Source: CAD feature listing. Evaluate the final solid. Frame: model axes, mm. A direction names the side the tool comes from. Give positions to 0.01 mm unless a question says otherwise; leave off trailing zeros. Write each loop counter-clockwise with the first axis right and the second up, starting at its lowest first coordinate (ties: lowest second). Pieces come first, ordered by that corner, then holes. Notation, with made-up numbers: (46.5, 80.25) -> (100.5, 80.25) arc R34 ccw to (100.5, 116.25) -> close; hole circle Ø11 at (60.5, 66.5). An arc over 180 degrees is marked (long way). Answer as a JSON object with one key per item and string values. Group by question number.
Item 1: Ray query, probe 1 along Y at (x, z) = (3.5, -11) (3 decimals); probe 2 along Z at (x, y) = (5.5, -1.25) (3 decimals); probe 3 along Y at (x, z) = (2.5, -16.5). Return the intervals inside material, ascending. Write a range as from..to.
Item 2: First-contact query: pin 1 Ø2 at (x, z) = (1.5, 6) entering from +Y (3 decimals); pin 2 Ø10 at (x, y) = (2, 9) entering from +Z (3 decimals). Flat tips, straight axial feed; report the tip coordinate or a pass-through.
Item 3: Access query for faces 4 (the face through (3.175, 2, -17)), 5 (the face through (9.525, -11, 2)), 6 (the face through (12.7, -10, -7)), 7 (the face through (-6, 3, -15.875)), 8 (the face through (0, -12.7, 0)). Directions: +Z, -Z, +X, -X, +Y, -Y. A direction counts if a zero-diameter tool reaches every point of the face in a straight line with its end or side. Return the directions, or none.
Item 4: Section query B-B on y = -1.5. Return the cut outline in (x, z) (3 decimals).
Item 5: Pull-direction query (X, two-part tool) for faces 1 (the face through (-12.7, -10, -7)), 2 (the face through (-0.07, -6.03, -17.44)), 3 (the face through (5, 0, -19.05)); classes: pulls with the +X half, pulls with the -X half, needs draft (parallel to the pull), parting line crosses it, or undercut.
Item 6: Section query A-A on x = 6.35. Return the cut outline in (y, z) (3 decimals).
Item 7: Section query C-C on z = -5. Return the cut outline in (x, y) (3 decimals), plus the area to 3 significant figures.
from build123d import *

# Parameters (mm, degrees)
BOSS_EXTRUDE1_DEPTH      = 12.7
BOSS_EXTRUDE1_DEPTH_BACK = 12.7
CUT_EXTRUDE1_DEPTH       = 40.272581084
CUT_EXTRUDE2_DEPTH       = 38.1
FILLET1_R                = 2.54


with BuildPart() as part:
    # Sketch2 → Boss-Extrude1 (new, two sides: drawn at the far end of the back side and taken through both)
    with BuildSketch(Plane(origin=(0, 0, 0), x_dir=(0, 0, -1), z_dir=(1, 0, 0)).offset(-BOSS_EXTRUDE1_DEPTH_BACK)):
        Polygon((15.875, -9.525), (-19.05, -9.525), (-19.05, -12.7), (19.05, -12.7), (19.05, 12.7), (15.875, 12.7), align=None)
    extrude(amount=BOSS_EXTRUDE1_DEPTH + BOSS_EXTRUDE1_DEPTH_BACK)

    # Sketch4 → Cut-Extrude1 (cut, through all)
    with BuildSketch(Plane.XY.offset(-15.875)):
        with BuildLine():
            Line((-3.175, 6.0325), (-3.175, -2.8575))
            ThreePointArc((-3.175, -2.8575), (0, -6.0325), (3.175, -2.8575))
            Line((3.175, -2.8575), (3.175, 6.0325))
            ThreePointArc((3.175, 6.0325), (0, 9.2075), (-3.175, 6.0325))
        make_face()
    extrude(amount=-CUT_EXTRUDE1_DEPTH, mode=Mode.SUBTRACT)

    # Sketch5 → Cut-Extrude2 (cut)
    with BuildSketch(Plane(origin=(0, -9.525, 0), x_dir=(1, 0, 0), z_dir=(0, 1, 0))):
        with BuildLine():
            Line((-3.175, 8.89), (-3.175, -12.065))
            ThreePointArc((-3.175, -12.065), (-6.35, -15.24), (-9.525, -12.065))
            Line((-9.525, -12.065), (-9.525, 8.89))
            ThreePointArc((-9.525, 8.89), (-6.35, 12.065), (-3.175, 8.89))
        make_face()
        with BuildLine():
            Line((3.175, 8.89), (3.175, -12.065))
            ThreePointArc((3.175, -12.065), (6.35, -15.24), (9.525, -12.065))
            Line((9.525, -12.065), (9.525, 8.89))
            ThreePointArc((9.525, 8.89), (6.35, 12.065), (3.175, 8.89))
        make_face()
    extrude(amount=-CUT_EXTRUDE2_DEPTH, mode=Mode.SUBTRACT)

    # Fillet1
    fillet1_edges = [part.edges().sort_by_distance(p)[0] for p in [
        (0, -9.525, -15.875),
    ]]
    fillet(fillet1_edges, radius=FILLET1_R)


solid = part.part
Worked answers:
{
 "1": {"probe 1": "-12.7..-9.525", "probe 2": "-19.05..-15.875", "probe 3": "-12.7..-4.81, 7.99..12.7"},
 "2": {"pin 1": "y = -9.525", "pin 2": "z = -15.875"},
 "3": {"face 4": "+Z, -Z", "face 5": "+Y, -Y", "face 6": "+Z, -Z, +X, +Y, -Y", "face 7": "+Z, +X, -X, +Y", "face 8": "+Z, -Z, +X, -X, -Y"},
 "4": {"outline": "(-12.7, -19.05) -> (-3.175, -19.05) -> (-3.175, -15.875) -> (-12.7, -15.875) -> close; (3.175, -19.05) -> (12.7, -19.05) -> (12.7, -15.875) -> (3.175, -15.875) -> close"},
 "5": {"face 1": "pulls with the -X half", "face 2": "undercut", "face 3": "needs draft"},
 "6": {"outline": "(-12.7, -19.05) -> (12.7, -19.05) -> (12.7, -15.875) -> (-6.985, -15.875) arc R2.54 cw to (-9.525, -13.335) -> (-9.525, -12.065) -> (-12.7, -12.065) -> close; (-12.7, 15.24) -> (-9.525, 15.24) -> (-9.525, 19.05) -> (-12.7, 19.05) -> close"},
 "7": {"outline": "(-12.7, -12.7) -> (-9.525, -12.7) -> (-9.525, -9.525) -> (-12.7, -9.525) -> close; (-3.175, -12.7) -> (3.175, -12.7) -> (3.175, -9.525) -> (-3.175, -9.525) -> close; (9.525, -12.7) -> (12.7, -12.7) -> (12.7, -9.525) -> (9.525, -9.525) -> close", "area": "40.3 mm^2"}
}
